Model file for the job. Use its own axes, mm. Face numbers are marked on the shaded views. A direction names the side the tool comes from. Coordinates: 2 decimals unless noted, no trailing zeros. Order: outer loops, then holes, each group sorted by start corner. A loop starts at its lowest first (then second) coordinate and runs counter-clockwise, first axis right, second up. Notation, with made-up numbers: M 74.25,-20.75 L 127.25,-20.75 A15 cw 127.25,-4.75 Z; hole C 87.25,-4 d7. An arc over 180 degrees is marked long. Return JSON: item names as keys, results as strings.
Autodesk Inventor part; units mm, degrees
ref_plane "YZ Plane" through (0, 0, 0) normal (1, 0, 0) x (0, 1, 0)
ref_plane "XZ Plane" through (0, 0, 0) normal (0, 1, 0) x (-1, 0, 0)
sketch "Sketch1" plane through (0, 0, 0) normal (0, 1, 0) x (-1, 0, 0)
  line L0 (0, 0) -> (-28, 0)
  line L1 (-28, 0) -> (-28, 16)
  line L2 (-28, 16) -> (0, 16)
  line L3 (0, 16) -> (0, 0)
  circle A0 centre (-25.1, 13.15) radius 1.5
  circle A1 centre (-2.9, 2.85) radius 1.5
  line L4 (-28, 8) -> (0, 8) construction
  line L5 (-14, 0) -> (-14, 16) construction
  line L6 (-25.1, 13.15) -> (-28, 13.15) construction
  line L7 (-25.1, 13.15) -> (-25.1, 16) construction
  line L8 (-2.9, 2.85) -> (-2.9, 0) construction
  line L9 (-2.9, 2.85) -> (0, 2.85) construction
  dimension "d0" = 28
  dimension "d1" = 16
  dimension "d2" = 3
  dimension "d3" = 3
  dimension "d4" = 22.2
  dimension "d5" = 10.3
extrude "Extrusion1" add sketch "Sketch1" along normal blind 10.2
ref_plane "Work Plane1" through (0, 0, 4.5) normal (0, 0, 1) x (1, 0, 0)
sketch "Sketch2" plane through (0, 0, 4.5) normal (0, 0, 1) x (1, 0, 0)
  line L0 (28, 1.925) -> (33.5, 1.925)
  line L1 (33.5, 1.925) -> (33.5, 2.8)
  line L2 (33.5, 8.275) -> (28, 8.275)
  line L3 (28, 8.275) -> (28, 1.925)
  line L4 (33.5, 7.4) -> (40, 7.4)
  line L5 (40, 7.4) -> (40, 2.8)
  line L6 (40, 2.8) -> (33.5, 2.8)
  line L7 (33.5, 7.4) -> (33.5, 8.275)
  line L8 (33.5, 2.8) -> (33.5, 7.4) construction
  line L9 (28, 1.925) -> (28, 0) construction
  line L10 (28, 8.275) -> (28, 10.2) construction
  circle A0 centre (38, 5.1) radius 0.85
  line L11 (38, 5.1) -> (38, 2.8) construction
  line L12 (38, 7.4) -> (38, 5.1) construction
  point P0 (0, 0)
  dimension "d12" = 6.5
  dimension "d13" = 1.7
  dimension "d14" = 2
  dimension "d15" = 12
  dimension "d16" = 4.6
  dimension "d17" = 6.35
extrude "Extrusion2" add sketch "Sketch2" along normal blind 0.8
ref_plane "Work Plane2" through (0, 1, 0) normal (0, -1, 0) x (1, 0, 0)
sketch "Sketch4" plane through (0, 1, 0) normal (0, -1, 0) x (1, 0, 0)
  line L0 (16.8061, 0) -> (16, 0)
  line L1 (16, 0) -> (16, -2.2)
  line L2 (16.8, -3) -> (16.8, -3)
  line L3 (16.8, -3) -> (26.1061, -3)
  line L4 (26.1061, -3) -> (26.1061, -2.2)
  line L5 (26.1061, -2.2) -> (17.6061, -2.2)
  line L6 (16.8061, -1.4) -> (16.8061, 0)
  arc A0 (16, -2.2) -> (16.8, -3) centre (16.8, -2.2) ccw
  arc A1 (16.8061, -1.4) -> (17.6061, -2.2) centre (17.6061, -1.4) ccw
  line L7 (0, 0) -> (0, 16)
  point P0 (16, -3)
  point P1 (16.8061, -2.2)
  dimension "d32" = 0.8
  dimension "d33" = 3
  dimension "d34" = 9.3
  dimension "d35" = 0.8
  dimension "d36" = 0.8
  dimension "d41" = 16
extrude "Extrusion3" add sketch "Sketch4" against normal blind 8.5
properties part number "game-switch"
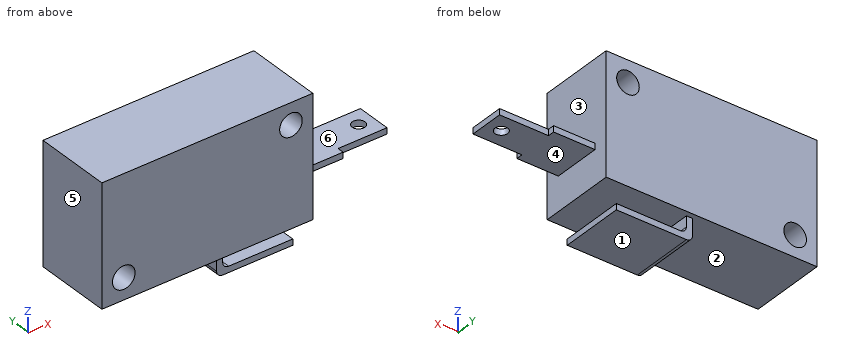
Item 1: 3-axis set-ups, long thin cutter, end or side, ignore diameter. For the marked faces 4, 5 and 6: which of +Z, -Z, +X, -X, +Y, -Y reach the whole face in a straight line?
Check result:
{"face 4": "-Z, +X, +Y, -Y", "face 5": "+Z, -Z, -X, +Y, -Y", "face 6": "+Z, +X, +Y, -Y"}
Item 2: Saw through at A-A (y = 5.1). Write the cut outline in (x, z).
Check result:
{"outline": "M 0,0 L 16,0 L 16,-2.2 A0.8 ccw 16.8,-3 L 26.11,-3 L 26.11,-2.2 L 17.61,-2.2 A0.8 cw 16.81,-1.4 L 16.81,0 L 28,0 L 28,4.5 L 37.15,4.5 L 37.15,5.3 L 28,5.3 L 28,16 L 0,16 Z; M 38.85,4.5 L 40,4.5 L 40,5.3 L 38.85,5.3 Z; hole C 2.9,2.85 d3; hole C 25.1,13.15 d3"}
Item 3: Drop flat-ended pins along their axis: pin 1 Ø2 at (x, z) = (21, 6) entering from -Y; pin 2 Ø2.5 at (x, z) = (2.9, 2.85) entering from +Y; pin 3 Ø1.1 at (y, z) = (4, -1) entering from -X; pin 4 Ø2 at (x, y) = (30, 3.5) entering from +Z. Give the stop position or say it passes through.
Check result:
{"pin 1": "stops at y = 0", "pin 2": "passes through", "pin 3": "stops at x = 16", "pin 4": "stops at z = 5.3"}
Item 4: Saw through at B-B (x = 38). Write the cut outline in (y, z), and give its area (3 significant figures).
Check result:
{"outline": "M 2.8,4.5 L 4.25,4.5 L 4.25,5.3 L 2.8,5.3 Z; M 5.95,4.5 L 7.4,4.5 L 7.4,5.3 L 5.95,5.3 Z", "area": "2.32 mm2"}
Item 5: Saw through at C-C (z = 13.15). Write the cut outline in (x, y), and give its area (3 significant figures).
Check result:
{"outline": "M 0,0 L 23.6,0 L 23.6,10.2 L 0,10.2 Z; M 26.6,0 L 28,0 L 28,10.2 L 26.6,10.2 Z", "area": "255 mm2"}
Item 6: Saw through at D-D (y = 9). Write the cut outline in (x, z).
Check result:
{"outline": "M 0,0 L 16,0 L 16,-2.2 A0.8 ccw 16.8,-3 L 26.11,-3 L 26.11,-2.2 L 17.61,-2.2 A0.8 cw 16.81,-1.4 L 16.81,0 L 28,0 L 28,16 L 0,16 Z; hole C 2.9,2.85 d3; hole C 25.1,13.15 d3"}
Item 7: Pull direction Z, two halves, no side cores. Call the marked faces 1, 2 and 3: +Z half, -Z half, draft (parallel to the pull), parting line (faces both ways), or undercut.
Check result:
{"face 1": "-Z half", "face 2": "undercut", "face 3": "draft"}
Item 8: Wall check: line 1 (Z direction, x = 25.1, y = 6.25); line 2 (Z direction, x = 34, y = 6.5); line 3 (Z direction, x = 10.5, y = 1.25). Give the ranges that are in metal, low to high.
Check result:
{"line 1": "z = -3 to -2.2, 0 to 11.65, 14.65 to 16", "line 2": "z = 4.5 to 5.3", "line 3": "z = 0 to 16"}
